Model file for the job. Use its own axes, mm. A direction names the side the tool comes from. Coordinates: 2 decimals unless noted, no trailing zeros. Loops run counter-clockwise (first coordinate to the right, second up) from the corner with the lowest first, then second, coordinate; pieces in that order, holes last.
from build123d import *

# Parameters (mm, degrees)
MODEL_R                 = 1.5
SALIENTE_EXTRUIR1_DEPTH = 3


with BuildPart() as part:
    # Model → Saliente-Extruir1 (new body)
    with BuildSketch(Plane.XY):
        with BuildLine():
            Line((363.137702798, 192.955720999), (379.819683313, 176.273740484))
            ThreePointArc((379.819683313, 176.273740484), (386.183644344, 176.273740484), (386.183644344, 182.637701515))
            Line((386.183644344, 182.637701515), (368.183644344, 200.637701515))
            ThreePointArc((368.183644344, 200.637701515), (366.723739274, 201.613178895), (365.001663828, 201.955720999))
            Line((365.001663828, 201.955720999), (348.865624859, 201.955720999))
            Line((348.865624859, 201.955720999), (341.183644344, 209.637701515))
            ThreePointArc((341.183644344, 209.637701515), (334.819683313, 209.637701515), (334.819683313, 203.273740484))
            Line((334.819683313, 203.273740484), (343.819683313, 194.273740484))
            ThreePointArc((343.819683313, 194.273740484), (345.279588383, 193.298263103), (347.001663828, 192.955720999))
            Line((347.001663828, 192.955720999), (363.137702798, 192.955720999))
        make_face()
        with Locations((356.001663828, 197.455720999)):
            Circle(MODEL_R, mode=Mode.SUBTRACT)
        with Locations((365.001663828, 197.455720999)):
            Circle(MODEL_R, mode=Mode.SUBTRACT)
        with Locations((383.001663828, 179.455720999)):
            Circle(MODEL_R, mode=Mode.SUBTRACT)
        with Locations((374.001663828, 188.455720999)):
            Circle(MODEL_R, mode=Mode.SUBTRACT)
        with Locations((347.001663828, 197.455720999)):
            Circle(MODEL_R, mode=Mode.SUBTRACT)
        with Locations((338.001663828, 206.455720999)):
            Circle(MODEL_R, mode=Mode.SUBTRACT)
    extrude(amount=SALIENTE_EXTRUIR1_DEPTH)


solid = part.part
Q1. Drill centre lines: line 1 (Y direction, x = 352, z = 2.5); line 2 (Y direction, x = 356.5, z = 1.15); line 3 (Y direction, x = 346.5, z = 0.95). Where is each one in solid material? Low to high.
Answers:
line 1: y = 192.96 to 201.96
line 2: y = 192.96 to 196.04, 198.87 to 201.96
line 3: y = 192.98 to 196.04, 198.87 to 204.32
Q2. Mould opens along Y. For faces 4 (the cylindrical face through (334.89, 209.707, 1.479)), 5 (the cylindrical face through (354.896, 198.469, 1.479)), 6 (the cylindrical face through (345.257, 193.308, 1.479)), 7 (the flat face through (345.08, 205.74, 1.48)) say: +Y half, -Y half, draft (parallel to the pull), parting line (faces both ways), or undercut.
Answers:
face 4: parting line
face 5: undercut
face 6: -Y half
face 7: +Y half
Q3. Slice it at A-A (x = 383). List the corners of the cut face in (y, z).
Answers:
outline: (174.96, 0) - (177.96, 0) - (177.96, 3) - (174.96, 3) - close; (180.96, 0) - (185.82, 0) - (185.82, 3) - (180.96, 3) - close
Q4. Slice it at B-B (z = 1.8). List the corners of the cut face in (x, y), and give its area (3 significant figures).
Answers:
outline: (334.82, 203.27) - (343.82, 194.27) arc R4.5 ccw to (347, 192.96) - (363.14, 192.96) - (379.82, 176.27) arc R4.5 ccw to (386.18, 182.64) - (368.18, 200.64) arc R4.5 ccw to (365, 201.96) - (348.87, 201.96) - (341.18, 209.64) arc R4.5 ccw to start; hole circle Ø3 at (338, 206.46); hole circle Ø3 at (347, 197.46); hole circle Ø3 at (356, 197.46); hole circle Ø3 at (365, 197.46); hole circle Ø3 at (374, 188.46); hole circle Ø3 at (383, 179.46)
area: 526 mm2
Q5. Slice it at C-C (x = 355.5). List the corners of the cut face in (y, z).
Answers:
outline: (192.96, 0) - (196.04, 0) - (196.04, 3) - (192.96, 3) - close; (198.87, 0) - (201.96, 0) - (201.96, 3) - (198.87, 3) - close
Q6. Which spindle directions (+Z, -Z, +X, -X, +Y, -Y) get a long thin tool onto all of the face, cutting with end or side? Do faces 1 (the flat face through (355, 192.956, 1)), 2 (the cylindrical face through (386.11, 176.2, 1.48)), 3 (the flat face through (357, 201.956, 1)). Say none if no direction does.
Answers:
face 1: +Z, -Z, -X, -Y
face 2: +Z, -Z
face 3: +Z, -Z, +X, +Y
Q7. Slice it at D-D (y = 202.5). List the corners of the cut face in (x, z), and give its area (3 significant figures).
Answers:
outline: (335.59, 0) - (348.32, 0) - (348.32, 3) - (335.59, 3) - close
area: 38.2 mm2
Q8. Flat gauge pin, fed straight in: P1, Ø1, axis at x = 381.5, z = 1, coming from the +Y side. Where does the tip first touch, or does it go through?
Answers:
P1: stops at y = 187.82
